from build123d import *

# Parameters (mm, degrees)
F0_W     = 304.8
F0_H     = 203.2
F1_DEPTH = 25.4
F2_R     = 3.175
F3_DEPTH = 25.4


with BuildPart() as f1:
    # F0 (on Front) → F1 (new body)
    with BuildSketch(Plane.XZ):
        with Locations((-3.048005, 2.967953)):
            Rectangle(F0_W, F0_H)
    extrude(amount=F1_DEPTH)

    # F2 (on face) → F3 (join)
    with BuildSketch(Plane.XZ.offset(25.4)):
        with Locations((-53.848005, -73.232047)):
            Circle(F2_R)
        with Locations((-107.806627, -43.933121)):
            Circle(F2_R)
    extrude(amount=F3_DEPTH)

    # F4 (on face) → F5 (revolve, cut)
    with BuildSketch(Plane.XZ.offset(25.4)):
        Polygon((149.351995, 16.831879), (-155.448005, 16.831879), (-155.448005, -2.218121), (-76.879319, -2.218121), (149.351995, -2.218121), align=None)
    revolve(axis=Axis((-3.048005, -25.4, 16.831879), (1, 0, 0)), mode=Mode.SUBTRACT)


solid = f1.part
Input: part model. Units: mm. Frame: model coordinates. A direction names the side the tool comes from. Give positions to 0.01 mm unless a question says otherwise; leave off trailing zeros. Order: outer loops, then holes, each group sorted by start corner. A loop starts at its lowest first (then second) coordinate and runs counter-clockwise, first axis right, second up. Notation, with made-up numbers: (8.5, 0.25) - (64.5, 0.25) arc R21 cw to (64.5, 26.25) - close; hole circle Ø3 at (41, 55.5). An arc over 180 degrees is marked (long way). Answer as a JSON object with one key per item and string values. Group by question number.
Q1. Cut plane C-C, the plane z = -16.5. Output: boundary loops of the cut face in (x, y).
Q2. Set-up query: faces 4 (the face through (-110.3, -37.9, -45.9)), 5 (the face through (-155.448, -13, 2)). Return all of +Z, -Z, +X, -X, +Y, -Y with unobstructed straight access to the full face (end or side cutting, diameter ignored); none if empty.
Q3. Cut plane A-A, the plane y = -14. Output: boundary loops of the cut face in (x, z), then the cut area to 3 significant figures.
Q4. Cut plane B-B, the plane x = 87. Output: boundary loops of the cut face in (y, z).
Q5. First-contact query: pin 1 Ø1 at (x, z) = (-3, -70.5) entering from +Y; pin 2 Ø10 at (y, z) = (-26.5, 27) entering from +X; pin 3 Ø1.5 at (x, z) = (-35, 81.5) entering from -Y. Flat tips, straight axial feed; report the tip coordinate or a pass-through.
Q6. Cut plane D-D, the plane y = -37.5. Output: boundary loops of the cut face in (x, z) (3 decimals), then the cut area to 3 significant figures.
Q7. Line query: probe 1 along Z at (x, y) = (95, -24); probe 2 along Z at (x, y) = (-82.5, -25); probe 3 along Y at (x, z) = (49, -13). Output: solid intervals per line, ascending.
Q8. Mould query, pull axis Z, two halves, no side actions, for faces 1 (the face through (-0.914, -6.355, 16.413)), 2 (the face through (149.352, -13, 2)), 3 (the face through (-5, -13, -98.632)). Classes: pulls with the +Z half, pulls with the -Z half, needs draft (parallel to the pull), parting line crosses it, or undercut.
Results:
{
 "1": {"outline": "(-155.45, -25.4) - (149.35, -25.4) - (149.35, 0) - (-155.45, 0) - close"},
 "2": {"face 4": "-Y", "face 5": "+Z, -Z, -X, +Y, -Y"},
 "3": {"outline": "(-155.45, -98.63) - (149.35, -98.63) - (149.35, 1.57) - (-155.45, 1.57) - close; (-155.45, 32.09) - (149.35, 32.09) - (149.35, 104.57) - (-155.45, 104.57) - close", "area": "52,600 mm^2"},
 "4": {"outline": "(-25.4, -98.63) - (0, -98.63) - (0, 104.57) - (-25.4, 104.57) - (-25.4, 35.88) arc R19.05 cw to (-25.4, -2.22) - close"},
 "5": {"pin 1": "y = 0", "pin 2": "through", "pin 3": "y = -25.4"},
 "6": {"outline": "circle Ø6.35 at (-107.807, -43.933); circle Ø6.35 at (-53.848, -73.232)", "area": "63.3 mm^2"},
 "7": {"probe 1": "-98.63 to -2.17, 35.83 to 104.57", "probe 2": "-98.63 to -2.21, 35.88 to 104.57", "probe 3": "-25.4 to 0"},
 "8": {"face 1": "undercut", "face 2": "needs draft", "face 3": "pulls with the -Z half"}
}
